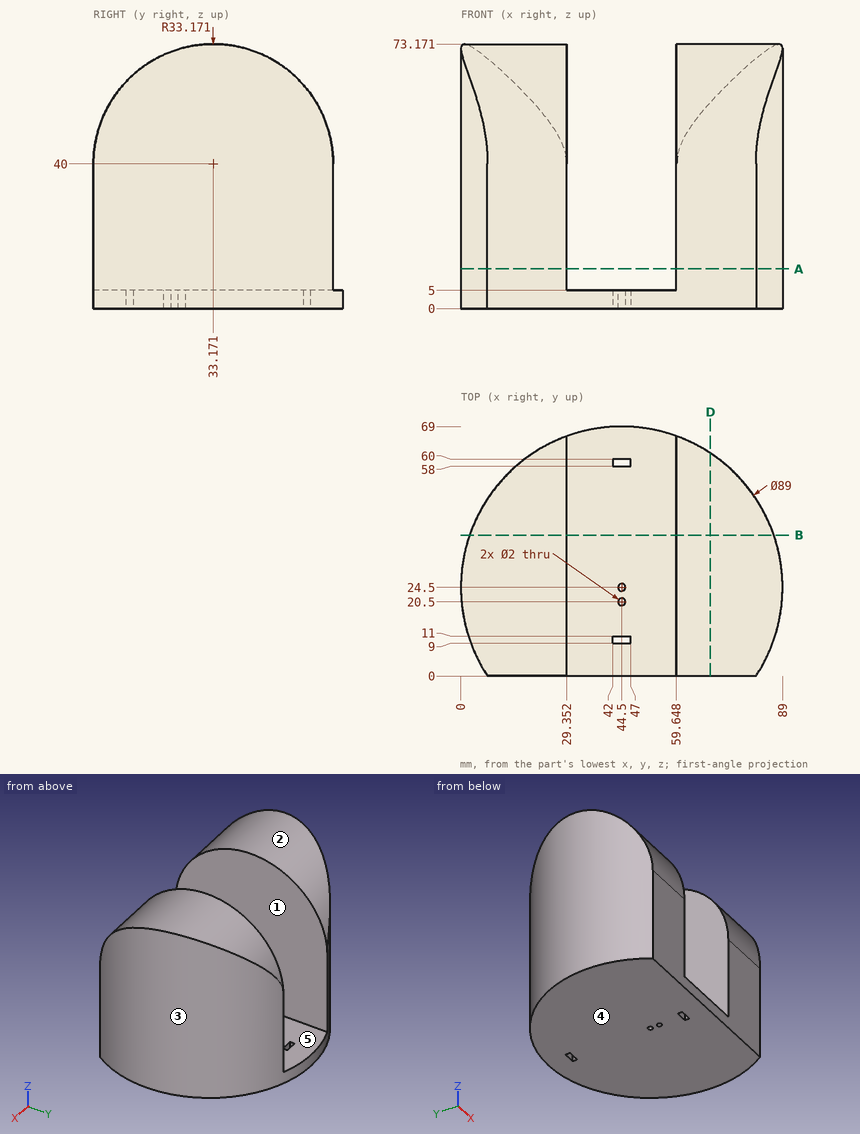
Here's the drawing with two shaded views (mm, measured from the low corner). I have some questions. A direction names the side the tool comes from. Give positions to 0.01 mm unless a question says otherwise; leave off trailing zeros. Loops run counter-clockwise (first coordinate to the right, second up) from the corner with the lowest first, then second, coordinate; pieces in that order, holes last. Notation, with made-up numbers: M 28.25,36.5 L 76.25,36.5 A16 cw 76.25,41.5 Z; hole C 16,11.25 d5. An arc over 180 degrees is marked long. Answer in a Markdown table with one row per item.
1. Suppose I cut it at D-D on x = 69. Write out the boundary of the cut face in (y, z).
Taken from the geometry:
| item | result |
|---|---|
| outline | M 0,0 L 61.65,0 L 61.65,57.01 A33.17 ccw 0,40 Z |
2. If I drill on line 1 along X through (y, z) = (10, 51); line 2 along X through (y, z) = (18, 13); line 3 along Z through (x, y) = (36.5, 24), over which ranges is the centre line in solid material (lowest first)?
Taken from the geometry:
| item | result |
|---|---|
| line 1 | x = 2.43 to 29.35, 59.65 to 86.57 |
| line 2 | x = 0.48 to 29.35, 59.65 to 88.52 |
| line 3 | z = 0 to 5 |
3. Which directions (+Z, -Z, +X, -X, +Y, -Y) give clear straight access to the entire face, cutting with the end or side of a thin tool? Please do the marked faces 1 and 2.
Taken from the geometry:
| item | result |
|---|---|
| face 1 | +Z, +Y, -Y |
| face 2 | +Z, +X, -X |
4. For pin 1 Ø1.6 at (y, z) = (10.5, 3.5) entering from -X; pin 2 Ø1.5 at (y, z) = (15, 43) entering from -X; pin 3 Ø0.6 at (y, z) = (58.5, 2.5) entering from +X, each with a flat end and sliding along its axis, tell me the tip position at first contact or that it passes through.
Taken from the geometry:
| item | result |
|---|---|
| pin 1 | stops at x = 2 |
| pin 2 | stops at x = 0.87 |
| pin 3 | stops at x = 73.56 |
5. Suppose I cut it at B-B on y = 39. Write out the boundary of the cut face in (x, z) (1 decimal), plus the area to 3 significant figures.
Taken from the geometry:
| item | result |
|---|---|
| outline | M 2.4,0 L 86.6,0 L 86.6,72.7 L 59.6,72.7 L 59.6,5 L 29.4,5 L 29.4,72.7 L 2.4,72.7 Z |
| area | 4,060 mm² |
6. Suppose I cut it at A-A on z = 11. Write out the boundary of the cut face in (x, y), plus the area to 3 significant figures.
Taken from the geometry:
| item | result |
|---|---|
| outline | M 7.35,0 L 29.35,0 L 29.35,66.34 A44.5 ccw Z; M 59.65,0 L 81.65,0 A44.5 ccw 59.65,66.34 Z |
| area | 3,110 mm² |
7. Thinking about a two-plate mould opening in X: for the marked faces 3, 4 and 5, which applies, released by +X, released by -X, zero draft, split by the parting line, or undercut?
Taken from the geometry:
| item | result |
|---|---|
| face 3 | split by the parting line |
| face 4 | zero draft |
| face 5 | undercut |
